from build123d import *

# Parameters (mm, degrees)
SKETCH2_W           = 35
SKETCH2_H           = 125
SKETCH2_W_2         = 11
SKETCH2_H_2         = 101
BOSS_EXTRUDE1_DEPTH = 850
SKETCH3_R           = 6
CUT_EXTRUDE1_DEPTH  = 860.854638878
SKETCH4_W           = 250
SKETCH4_H           = 150
BOSS_EXTRUDE2_DEPTH = 12
SKETCH5_W           = 250
SKETCH5_H           = 150
BOSS_EXTRUDE3_DEPTH = 12
BOSS_EXTRUDE4_START = -62.5
BOSS_EXTRUDE4_DEPTH = 6
SKETCH8_R           = 6
CUT_EXTRUDE2_DEPTH  = 12


with BuildPart() as part:
    # Sketch2 → Boss-Extrude1 (new body)
    with BuildSketch(Plane(origin=(0, 0, 0), x_dir=(1, 0, 0), z_dir=(0, 1, 0))):
        with Locations((17.5, 62.5)):
            Rectangle(SKETCH2_W, SKETCH2_H)
        with Locations((17.5, 62.5)):
            Rectangle(SKETCH2_W_2, SKETCH2_H_2, mode=Mode.SUBTRACT)
    extrude(amount=BOSS_EXTRUDE1_DEPTH)

    # Sketch3 → Cut-Extrude1 (cut, through all)
    with BuildSketch(Plane(origin=(35, 0, 0), x_dir=(0, 0, -1), z_dir=(1, 0, 0))):
        with Locations((62.5, 575)):
            Circle(SKETCH3_R)
        with Locations((62.5, 525)):
            Circle(SKETCH3_R)
        with Locations((105.801270189, 550)):
            Circle(SKETCH3_R)
        with Locations((37.5, 425)):
            Circle(SKETCH3_R)
        with Locations((87.5, 425)):
            Circle(SKETCH3_R)
        with Locations((105.801270189, 300)):
            Circle(SKETCH3_R)
        with Locations((62.5, 325)):
            Circle(SKETCH3_R)
        with Locations((62.5, 275)):
            Circle(SKETCH3_R)
    extrude(amount=-CUT_EXTRUDE1_DEPTH, mode=Mode.SUBTRACT)

    # Sketch4 → Boss-Extrude2 (add)
    with BuildSketch(Plane(origin=(0, 0, 0), x_dir=(-1, 0, 0), z_dir=(0, -1, 0))):
        with Locations((-17.5, 62.5)):
            Rectangle(SKETCH4_W, SKETCH4_H)
    extrude(amount=BOSS_EXTRUDE2_DEPTH)

    # Sketch5 → Boss-Extrude3 (add)
    with BuildSketch(Plane(origin=(0, 850, 0), x_dir=(1, 0, 0), z_dir=(0, 1, 0))):
        with Locations((17.5, 62.5)):
            Rectangle(SKETCH5_W, SKETCH5_H)
    extrude(amount=BOSS_EXTRUDE3_DEPTH)

    # Sketch7 → Boss-Extrude4 (add, symmetric)
    with BuildSketch(Plane(origin=(0, 0, -125), x_dir=(-1, 0, 0), z_dir=(0, 0, -1)).offset(BOSS_EXTRUDE4_START)):
        Polygon((-35, 0), (-35, 125), (-142.5, 0), align=None)
        Polygon((0, 125), (107.5, 0), (0, 0), align=None)
    extrude(amount=BOSS_EXTRUDE4_DEPTH, both=True)

    # Sketch8 → Cut-Extrude2 (cut)
    with BuildSketch(Plane(origin=(0, 0, 0), x_dir=(1, 0, 0), z_dir=(0, 1, 0))):
        with Locations(Location((-53.75, 28.25, 0), (0, 0, 270))):
            Circle(SKETCH8_R)
        with Locations(Location((-53.75, 96.75, 0), (0, 0, 270))):
            Circle(SKETCH8_R)
        with Locations(Location((88.75, 28.25, 0), (0, 0, 270))):
            Circle(SKETCH8_R)
        with Locations(Location((88.75, 96.75, 0), (0, 0, 270))):
            Circle(SKETCH8_R)
    extrude(amount=-CUT_EXTRUDE2_DEPTH, mode=Mode.SUBTRACT)


solid = part.part
Read the model definition and answer for the solid it produces. Units are mm, in the model's axes. A direction names the side the tool comes from. Give positions to 0.01 mm unless a question says otherwise; leave off trailing zeros. Loops run counter-clockwise (first coordinate to the right, second up) from the corner with the lowest first, then second, coordinate; pieces in that order, holes last. Notation, with made-up numbers: (43.5, 23.5) -> (70.5, 23.5) arc R9 cw to (70.5, 31.5) -> close; hole circle Ø7 at (31.5, 23.5). An arc over 180 degrees is marked (long way). Use a Markdown table: item, result.
Q1. Determine the mould class of faces 6 (the face through (88, 63.37, -62.42)), 7 (the face through (-53, 63.37, -62.58)), 8 (the face through (17, 419, 0)), 9 (the face through (23, 419, -62)) for opening direction X: pulls with the +X half, pulls with the -X half, needs draft (parallel to the pull), parting line crosses it, or undercut.
Solved:
| item | result |
|---|---|
| face 6 | pulls with the +X half |
| face 7 | pulls with the -X half |
| face 8 | needs draft |
| face 9 | undercut |
Q2. Section B-B, the plane x = -36.5 is taken. Determine the outline of the cut face in (y, z), then the cut area to 3 significant figures.
Solved:
| item | result |
|---|---|
| outline | (-12, -137.5) -> (0, -137.5) -> (0, -68.5) -> (82.56, -68.5) -> (82.56, -56.5) -> (0, -56.5) -> (0, 12.5) -> (-12, 12.5) -> close; (850, -137.5) -> (862, -137.5) -> (862, 12.5) -> (850, 12.5) -> close |
| area | 4,590 mm^2 |
Q3. Section A-A, the plane y = 140.5 is taken. Determine the outline of the cut face in (x, z).
Solved:
| item | result |
|---|---|
| outline | (0, -125) -> (35, -125) -> (35, 0) -> (0, 0) -> close; hole (12, -113) -> (23, -113) -> (23, -12) -> (12, -12) -> close |
Q4. Find the intervals of material crossed by line 1 along Z through (x, y) = (14.5, 303); line 2 along X through (y, z) = (60, -51.5); line 3 along Y through (x, z) = (-68.5, -111.5), in increasing order.
Solved:
| item | result |
|---|---|
| line 1 | z = -125 to -113, -12 to 0 |
| line 2 | x = 0 to 12, 23 to 35 |
| line 3 | y = -12 to 0, 850 to 862 |
Q5. Section C-C, the plane x = -75 is taken. Determine the outline of the cut face in (y, z).
Solved:
| item | result |
|---|---|
| outline | (-12, -137.5) -> (0, -137.5) -> (0, -68.5) -> (37.79, -68.5) -> (37.79, -56.5) -> (0, -56.5) -> (0, 12.5) -> (-12, 12.5) -> close; (850, -137.5) -> (862, -137.5) -> (862, 12.5) -> (850, 12.5) -> close |
Q6. A tool of negligible diameter and unlimited length cuts with its end or side. For faces 1 (the face through (66, 36, -68.5)), 2 (the face through (-31, 36, -56.5)), 3 (the face through (17, 419, -125)), 4 (the face through (19, 0, -126)), 5 (the face through (66, 36, -56.5)), from which of +Z, -Z, +X, -X, +Y, -Y can it reach the whole face along a straight path? Write none if from no direction.
Solved:
| item | result |
|---|---|
| face 1 | -Z, +X |
| face 2 | +Z, -X |
| face 3 | -Z, +X, -X |
| face 4 | -Z |
| face 5 | +Z, +X |
Q7. Each of these flat-tipped pins is pushed along its axis until it touches: pin 1 (6 mm diameter, centred on y = 636, z = -73, fed in from +X); pin 2 (7 mm diameter, centred on x = 88.75, z = -96.75, fed in from -Y); pin 3 (19 mm diameter, centred on y = 300, z = -105.8, fed in from -X). Where does it stop, or does it pass through?
Solved:
| item | result |
|---|---|
| pin 1 | stops at x = 35 |
| pin 2 | stops at y = 850 |
| pin 3 | stops at x = 0 |
